CAD build for the part. Positions are in the model's coordinates, mm. A direction names the side the tool comes from. Round coordinates to 2 decimals unless told otherwise and drop trailing zeros. Loops run counter-clockwise (first coordinate to the right, second up) from the corner with the lowest first, then second, coordinate; pieces in that order, holes last.
from build123d import *

# Parameters (mm, degrees)
BOSS_EXTRUDE1_DEPTH = 60
SKETCH2_R           = 7.5
CUT_EXTRUDE1_DEPTH  = 60
SKETCH3_R           = 5.25
CUT_EXTRUDE2_DEPTH  = 60
SKETCH4_R           = 11.5
CUT_EXTRUDE3_DEPTH  = 4
SKETCH5_W           = 10
SKETCH5_H           = 5
CUT_EXTRUDE4_DEPTH  = 60
SKETCH6_W           = 130
SKETCH6_H           = 90
BOSS_EXTRUDE2_DEPTH = 60
SKETCH8_W           = 130
SKETCH8_H           = 115
CUT_EXTRUDE6_DEPTH  = 20
SKETCH9_W           = 20.525641278
SKETCH9_H           = 90
CUT_EXTRUDE7_DEPTH  = 45
SKETCH7_R           = 38.5
CUT_EXTRUDE8_DEPTH  = 40
SKETCH12_W          = 88.948717444
SKETCH12_H          = 40
BOSS_EXTRUDE4_DEPTH = 7
SKETCH13_W          = 25
SKETCH13_H          = 40
BOSS_EXTRUDE5_DEPTH = 7
SKETCH14_W          = 25
SKETCH14_H          = 40
BOSS_EXTRUDE6_DEPTH = 7
SKETCH16_W          = 144.296296296
SKETCH16_H          = 122.248772368
CUT_EXTRUDE9_DEPTH  = 16
SKETCH23_R          = 10.574878896
BOSS_EXTRUDE7_DEPTH = 24
SKETCH24_R          = 5.3
CUT_EXTRUDE11_DEPTH = 24
SKETCH25_R          = 11.25
CUT_EXTRUDE12_DEPTH = 4
SKETCH26_R          = 41.241524366
BOSS_EXTRUDE8_DEPTH = 24
SKETCH27_R          = 38
CUT_EXTRUDE13_DEPTH = 24
FILLET2_R           = 30


with BuildPart() as part:
    # Sketch1 → Boss-Extrude1 (new body)
    with BuildSketch(Plane(origin=(0, 0, 0), x_dir=(1, 0, 0), z_dir=(0, 1, 0))):
        with BuildLine():
            Line((-65, 25), (65, 25))
            Line((65, 25), (65, -25))
            Line((65, -25), (32.897568299, -25))
            ThreePointArc((32.897568299, -25), (0, -6.5), (-32.897568299, -25))
            Line((-32.897568299, -25), (-65, -25))
            Line((-65, -25), (-65, 25))
        make_face()
    extrude(amount=BOSS_EXTRUDE1_DEPTH)

    # Sketch2 → Cut-Extrude1 (cut)
    with BuildSketch(Plane(origin=(0, 60, 0), x_dir=(1, 0, 0), z_dir=(0, 1, 0))):
        with Locations(Location((-51.452605548, 12.714222387, 0), (0, 0, 270))):
            Circle(SKETCH2_R)
        with Locations(Location((51.452605548, 12.714222387, 0), (0, 0, 90))):
            Circle(SKETCH2_R)
    extrude(amount=-CUT_EXTRUDE1_DEPTH, mode=Mode.SUBTRACT)

    # Sketch3 → Cut-Extrude2 (cut)
    with BuildSketch(Plane(origin=(0, 60, 0), x_dir=(1, 0, 0), z_dir=(0, 1, 0))):
        with Locations(Location((0, 12.714222387, 0), (0, 0, 270))):
            Circle(SKETCH3_R)
    extrude(amount=-CUT_EXTRUDE2_DEPTH, mode=Mode.SUBTRACT)

    # Sketch4 → Cut-Extrude3 (cut)
    with BuildSketch(Plane(origin=(0, 60, 0), x_dir=(1, 0, 0), z_dir=(0, 1, 0))):
        with Locations(Location((0, 12.714222387, 0), (0, 0, 270))):
            Circle(SKETCH4_R)
    extrude(amount=-CUT_EXTRUDE3_DEPTH, mode=Mode.SUBTRACT)

    # Sketch5 → Cut-Extrude4 (cut)
    with BuildSketch(Plane(origin=(0, 60, 0), x_dir=(1, 0, 0), z_dir=(0, 1, 0))):
        with Locations((-52.884181241, -16.580341224)):
            Rectangle(SKETCH5_W, SKETCH5_H)
        with Locations((-28.013085243, 17.079406564)):
            Rectangle(SKETCH5_W, SKETCH5_H)
        with Locations((52.884181241, -16.580341224)):
            Rectangle(SKETCH5_W, SKETCH5_H)
        with Locations((28.013085243, 17.079406564)):
            Rectangle(SKETCH5_W, SKETCH5_H)
    extrude(amount=-CUT_EXTRUDE4_DEPTH, mode=Mode.SUBTRACT)

    # Sketch6 → Boss-Extrude2 (add)
    with BuildSketch(Plane(origin=(0, 60, 0), x_dir=(1, 0, 0), z_dir=(0, 1, 0))):
        with Locations((0, -45)):
            Rectangle(SKETCH6_W, SKETCH6_H)
    extrude(amount=-BOSS_EXTRUDE2_DEPTH)

    # Sketch8 → Cut-Extrude6 (cut)
    with BuildSketch(Plane.XZ):
        with Locations((0, 32.5)):
            Rectangle(SKETCH8_W, SKETCH8_H)
    extrude(amount=-CUT_EXTRUDE6_DEPTH, mode=Mode.SUBTRACT)

    # Sketch9 → Cut-Extrude7 (cut)
    with BuildSketch(Plane(origin=(0, 60, 0), x_dir=(1, 0, 0), z_dir=(0, 1, 0))):
        with Locations((-54.737179361, -45)):
            Rectangle(SKETCH9_W, SKETCH9_H)
        with Locations((54.737179361, -45)):
            Rectangle(SKETCH9_W, SKETCH9_H)
    extrude(amount=-CUT_EXTRUDE7_DEPTH, mode=Mode.SUBTRACT)

    # Sketch7 → Cut-Extrude8 (cut)
    with BuildSketch(Plane(origin=(0, 60, 0), x_dir=(1, 0, 0), z_dir=(0, 1, 0))):
        with Locations(Location((0, -51.285777613, 0), (0, 0, 270))):
            Circle(SKETCH7_R)
    extrude(amount=-CUT_EXTRUDE8_DEPTH, mode=Mode.SUBTRACT)

    # Sketch12 → Boss-Extrude4 (add)
    with BuildSketch(Plane.XY.offset(90)):
        with Locations((0, 40)):
            Rectangle(SKETCH12_W, SKETCH12_H)
    extrude(amount=BOSS_EXTRUDE4_DEPTH)

    # Sketch13 → Boss-Extrude5 (add)
    with BuildSketch(Plane(origin=(65, 0, 0), x_dir=(0, 0, -1), z_dir=(1, 0, 0))):
        with Locations((12.5, 40)):
            Rectangle(SKETCH13_W, SKETCH13_H)
    extrude(amount=BOSS_EXTRUDE5_DEPTH)

    # Sketch14 → Boss-Extrude6 (add)
    with BuildSketch(Plane.ZY.offset(65)):
        with Locations((-12.5, 40)):
            Rectangle(SKETCH14_W, SKETCH14_H)
    extrude(amount=BOSS_EXTRUDE6_DEPTH)

    # Sketch16 → Cut-Extrude9 (cut)
    with BuildSketch(Plane(origin=(0, 60, 0), x_dir=(1, 0, 0), z_dir=(0, 1, 0))):
        with Locations((0.148148148, -36.124386184)):
            Rectangle(SKETCH16_W, SKETCH16_H)
    extrude(amount=-CUT_EXTRUDE9_DEPTH, mode=Mode.SUBTRACT)

    # Sketch23 → Boss-Extrude7 (add)
    with BuildSketch(Plane(origin=(0, 44, 0), x_dir=(1, 0, 0), z_dir=(0, 1, 0))):
        with Locations((0, 12.714222387)):
            Circle(SKETCH23_R)
    extrude(amount=-BOSS_EXTRUDE7_DEPTH)

    # Sketch24 → Cut-Extrude11 (cut)
    with BuildSketch(Plane(origin=(0, 44, 0), x_dir=(1, 0, 0), z_dir=(0, 1, 0))):
        with Locations(Location((0, 11.2, 0), (0, 0, 270))):
            Circle(SKETCH24_R)
    extrude(amount=-CUT_EXTRUDE11_DEPTH, mode=Mode.SUBTRACT)

    # Sketch25 → Cut-Extrude12 (cut)
    with BuildSketch(Plane(origin=(0, 44, 0), x_dir=(1, 0, 0), z_dir=(0, 1, 0))):
        with Locations(Location((0, 11.2, 0), (0, 0, 270))):
            Circle(SKETCH25_R)
    extrude(amount=-CUT_EXTRUDE12_DEPTH, mode=Mode.SUBTRACT)

    # Sketch26 → Boss-Extrude8 (add)
    with BuildSketch(Plane(origin=(0, 44, 0), x_dir=(1, 0, 0), z_dir=(0, 1, 0))):
        with Locations((0, -51.285777613)):
            Circle(SKETCH26_R)
    extrude(amount=-BOSS_EXTRUDE8_DEPTH)

    # Sketch27 → Cut-Extrude13 (cut)
    with BuildSketch(Plane(origin=(0, 44, 0), x_dir=(1, 0, 0), z_dir=(0, 1, 0))):
        with Locations(Location((0, -51.59650437, 0), (0, 0, 270))):
            Circle(SKETCH27_R)
    extrude(amount=-CUT_EXTRUDE13_DEPTH, mode=Mode.SUBTRACT)

    # Fillet2
    fillet2_edges = [part.edges().sort_by_distance(p)[0] for p in [
        (44.474358722, 32, 97),
        (-44.474358722, 32, 97),
    ]]
    fillet(fillet2_edges, radius=FILLET2_R)


solid = part.part
Item 1: Cut at D-D (y = 28.75). List the corners of the cut face in (x, z), plus the area to 3 significant figures.
Verdict:
outline: (-72, -25) - (72, -25) - (72, 0) - (44.47, 0) - (44.47, 67) arc R30 ccw to (14.47, 97) - (-14.47, 97) arc R30 ccw to (-44.47, 67) - (-44.47, 0) - (-72, 0) - close; hole circle Ø15 at (-51.45, -12.71); hole circle Ø76 at (0, 51.6); hole (-33.01, -19.58) - (-23.01, -19.58) - (-23.01, -14.58) - (-33.01, -14.58) - close; hole circle Ø10.6 at (0, -11.2); hole (23.01, -19.58) - (33.01, -19.58) - (33.01, -14.58) - (23.01, -14.58) - close; hole circle Ø15 at (51.45, -12.71)
area: 6,760 mm2
Item 2: Mould opens along Z. For faces 6 (the flat face through (0, 20, 13)), 7 (the flat face through (28, 32, -14.579)), 8 (the cylindrical face through (-35.9, 32.2, 88)) say: released by +Z, released by -Z, zero draft, split by the parting line, or undercut.
Verdict:
face 6: zero draft
face 7: undercut
face 8: released by +Z
Item 3: Cut at B-B (z = -11.2). List the corners of the cut face in (x, y), plus the area to 3 significant figures.
Verdict:
outline: (-72, 20) - (-58.8, 20) - (-58.8, 44) - (-72, 44) - close; (-44.11, 20) - (-5.3, 20) - (-5.3, 40) - (-11.25, 40) - (-11.25, 44) - (-44.11, 44) - close; (5.3, 20) - (44.11, 20) - (44.11, 44) - (11.25, 44) - (11.25, 40) - (5.3, 40) - close; (58.8, 20) - (72, 20) - (72, 44) - (58.8, 44) - close
area: 2,450 mm2
Item 4: Flat gauge pins, fed straight in: P1, Ø7, axis at y = 28.5, z = 29, coming from the -X side; P2, Ø9, axis at x = -51.45, z = -12.71, coming from the -Y side; P3, Ø11, axis at x = 4, z = -9, coming from the +Y side; P4, Ø2, axis at x = 48, y = 25, coming from the +Z side. Where does each tip first touch, or does it go through?
Verdict:
P1: stops at x = -44.47
P2: passes through
P3: stops at y = 40
P4: stops at z = 0
Item 5: 3-axis set-ups, long thin cutter, end or side, ignore diameter. For faces 1 (the flat face through (-23.013, 32, -17)), 2 (the flat face through (-72, 32, -13)), 3 (the flat face through (0, 44, 13)), 4 (the flat face through (-58, 32, 0)), 5 (the flat face through (44.474, 32, 33)): which of +Z, -Z, +X, -X, +Y, -Y reach the whole face in a straight line?
Verdict:
face 1: +Y, -Y
face 2: +Z, -Z, -X, +Y, -Y
face 3: +Z, -Z, +X, -X, +Y
face 4: +Z, -X, +Y, -Y
face 5: +Z, +X, +Y, -Y
Item 6: Cut at A-A (x = 0). List the corners of the cut face in (y, z).
Verdict:
outline: (20, -25) - (44, -25) - (44, -22.45) - (40, -22.45) - (40, -16.5) - (20, -16.5) - close; (20, -5.9) - (40, -5.9) - (40, 0.05) - (44, 0.05) - (44, 13.6) - (20, 13.6) - close; (20, 89.6) - (44, 89.6) - (44, 97) - (20, 97) - close
Item 7: Wall check: L1, parallel to X at y = 40.25, z = -17.5; L2, parallel to X at y = 25.5, z = -11.2; L3, parallel to X at y = 42, z = -11.2. Give the ranges that are in metal, low to high.
Verdict:
L1: x = -72 to -57.23, -45.68 to -33.01, -23.01 to -9.32, 9.32 to 23.01, 33.01 to 45.68, 57.23 to 72
L2: x = -72 to -58.8, -44.11 to -5.3, 5.3 to 44.11, 58.8 to 72
L3: x = -72 to -58.8, -44.11 to -11.25, 11.25 to 44.11, 58.8 to 72
Item 8: Cut at C-C (x = 57). List the corners of the cut face in (y, z), plus the area to 3 significant figures.
Verdict:
outline: (20, -25) - (44, -25) - (44, -17.76) - (20, -17.76) - close; (20, -7.67) - (44, -7.67) - (44, 0) - (20, 0) - close
area: 358 mm2
